from build123d import *

# Parameters (mm, degrees)
SKETCH1_W           = 70
SKETCH1_H           = 70
BOSS_EXTRUDE1_DEPTH = 42
SKETCH2_W           = 70
SKETCH2_H           = 70
BOSS_EXTRUDE2_DEPTH = 6
SKETCH3_R           = 4
CUT_EXTRUDE1_DEPTH  = 74
SKETCH6_W           = 10.07808718
SKETCH6_H           = 10.120371506
SKETCH6_W_2         = 10.137770901
SKETCH6_H_2         = 10.393985643
BOSS_EXTRUDE4_DEPTH = 28
FILLET1_R           = 1
SKETCH4_R           = 4.2
SKETCH4_R_2         = 3
BOSS_EXTRUDE3_DEPTH = 32
CUT_EXTRUDE2_START  = -28
SKETCH8_R           = 3
CUT_EXTRUDE2_DEPTH  = 28
FILLET2_R           = 1


with BuildPart() as part:
    # Sketch1 → Boss-Extrude1 (new body)
    with BuildSketch(Plane(origin=(0, 0, 0), x_dir=(1, 0, 0), z_dir=(0, 1, 0))):
        with Locations((22.315, -31.66)):
            Rectangle(SKETCH1_W, SKETCH1_H)
        with BuildLine():
            Line((1, 0), (43.63, 0))
            ThreePointArc((43.63, 0), (44.337106781, -0.292893219), (44.63, -1))
            Line((44.63, -1), (44.63, -62.32))
            ThreePointArc((44.63, -62.32), (44.337106781, -63.027106781), (43.63, -63.32))
            Line((43.63, -63.32), (1, -63.32))
            ThreePointArc((1, -63.32), (0.292893219, -63.027106781), (0, -62.32))
            Line((0, -62.32), (0, -1))
            ThreePointArc((0, -1), (0.292893219, -0.292893219), (1, 0))
        make_face(mode=Mode.SUBTRACT)
    extrude(amount=BOSS_EXTRUDE1_DEPTH)

    # Sketch2 → Boss-Extrude2 (add)
    with BuildSketch(Plane(origin=(0, 42, 0), x_dir=(1, 0, 0), z_dir=(0, 1, 0))):
        with Locations((22.315, -31.66)):
            Rectangle(SKETCH2_W, SKETCH2_H)
    extrude(amount=BOSS_EXTRUDE2_DEPTH)

    # Sketch3 → Cut-Extrude1 (cut)
    with BuildSketch(Plane.XY.offset(66.66)):
        with Locations((22.315, 33.289388907)):
            Circle(SKETCH3_R)
    extrude(amount=-CUT_EXTRUDE1_DEPTH, mode=Mode.SUBTRACT)

    # Sketch6 → Boss-Extrude4 (add)
    with BuildSketch(Plane(origin=(0, 42, 0), x_dir=(-1, 0, 0), z_dir=(0, -1, 0))):
        with Locations((-5.03904359, -58.259814247)):
            Rectangle(SKETCH6_W, SKETCH6_H)
        with Locations((-39.56111455, -58.259814247)):
            Rectangle(SKETCH6_W_2, SKETCH6_H)
        with Locations((-39.56111455, -5.196992822)):
            Rectangle(SKETCH6_W_2, SKETCH6_H_2)
        with Locations((-5.03904359, -5.196992822)):
            Rectangle(SKETCH6_W, SKETCH6_H_2)
    extrude(amount=BOSS_EXTRUDE4_DEPTH)

    # Fillet1
    fillet1_edges = [part.edges().sort_by_distance(p)[0] for p in [
        (34.492229099, 28, 10.393985643),
        (10.07808718, 28, 10.393985643),
        (10.07808718, 28, 53.199628494),
        (34.492229099, 28, 53.199628494),
    ]]
    fillet(fillet1_edges, radius=FILLET1_R)

    # Sketch4 → Boss-Extrude3 (add)
    # profile 1 of 4: a face of its own
    with BuildSketch(Plane.XZ.offset(-42)):
        with Locations(Location((5.703606864, 5.703606864, 0), (0, 0, 90))):
            Circle(SKETCH4_R)
        with Locations(Location((5.703606864, 5.703606864, 0), (0, 0, 90))):
            Circle(SKETCH4_R_2, mode=Mode.SUBTRACT)
    # profile 2 of 4: a face of its own
    with BuildSketch(Plane.XZ.offset(-42)):
        with Locations(Location((38.926393136, 5.703606864, 0), (0, 0, 270))):
            Circle(SKETCH4_R)
        with Locations(Location((38.926393136, 5.703606864, 0), (0, 0, 270))):
            Circle(SKETCH4_R_2, mode=Mode.SUBTRACT)
    # profile 3 of 4: a face of its own
    with BuildSketch(Plane.XZ.offset(-42)):
        with Locations(Location((38.926393136, 57.616393136, 0), (0, 0, 90))):
            Circle(SKETCH4_R)
        with Locations(Location((38.926393136, 57.616393136, 0), (0, 0, 90))):
            Circle(SKETCH4_R_2, mode=Mode.SUBTRACT)
    # profile 4 of 4: a face of its own
    with BuildSketch(Plane.XZ.offset(-42)):
        with Locations(Location((5.703606864, 57.616393136, 0), (0, 0, 270))):
            Circle(SKETCH4_R)
        with Locations(Location((5.703606864, 57.616393136, 0), (0, 0, 270))):
            Circle(SKETCH4_R_2, mode=Mode.SUBTRACT)
    extrude(amount=BOSS_EXTRUDE3_DEPTH)

    # Sketch8 → Cut-Extrude2 (cut)
    with BuildSketch(Plane(origin=(0, 14, 0), x_dir=(-1, 0, 0), z_dir=(0, -1, 0)).offset(CUT_EXTRUDE2_START)):
        with Locations(Location((-5.703606864, -57.616393136, 0), (0, 0, 90))):
            Circle(SKETCH8_R)
        with Locations(Location((-38.926393136, -57.616393136, 0), (0, 0, 90))):
            Circle(SKETCH8_R)
        with Locations(Location((-38.926393136, -5.703606864, 0), (0, 0, 90))):
            Circle(SKETCH8_R)
        with Locations(Location((-5.703606864, -5.703606864, 0), (0, 0, 90))):
            Circle(SKETCH8_R)
    extrude(amount=CUT_EXTRUDE2_DEPTH, mode=Mode.SUBTRACT)

    # Fillet2
    fillet2_edges = [part.edges().sort_by_distance(p)[0] for p in [
        (18.315, 33.289388907, 0),
        (18.315, 33.289388907, 63.32),
    ]]
    fillet(fillet2_edges, radius=FILLET2_R)


solid = part.part
Build history of the part. All positions in model axes, mm. A direction names the side the tool comes from. Coordinates: 2 decimals unless noted, no trailing zeros. Write each loop counter-clockwise with the first axis right and the second up, starting at its lowest first coordinate (ties: lowest second). Pieces come first, ordered by that corner, then holes. Notation, with made-up numbers: (2.5, 72.25) -> (17.5, 72.25) arc R28 ccw to (17.5, 102.25) -> close; hole circle Ø7 at (-26, 25.25). An arc over 180 degrees is marked (long way). Use CSV: the item, a comma, the result in double quotes. Start each with the question number.
Q1. Cut at A-A, the plane y = 11. State how many separate pieces and enclosed holes the cut face has, then the cut area to 3 significant figures.
Q2. Cut at C-C, the plane x = 12. List the corners of the cut face in (y, z), then the cut area to 3 significant figures.
Q3. Pull direction Y, two halves, no side cores. Call faces 1 (the flat face through (0, 21, 32)), 2 (the flat face through (9, 10, 59)), 3 (the cylindrical face through (19.141, 30.855, -2.154)): released by +Y, released by -Y, zero draft, split by the parting line, or undercut.
Q4. Drill centre lines: probe 1 along Z at (x, y) = (4, 29.5); probe 2 along X at (y, z) = (41, 0.5) (3 decimals); probe 3 along X at (y, z) = (40.5, 18.5) (3 decimals). Where is each one in solid material? Low to high.
Q5. Cut at D-D, the plane y = 22. List the corners of the cut face in (x, z) (3 decimals).
Q6. Cut at B-B, the plane z = 51.5. List the corners of the cut face in (x, y) (3 decimals).
Q7. 3-axis set-ups, long thin cutter, end or side, ignore diameter. For faces 4 (the flat face through (-12.685, 24, 32)), 5 (the flat face through (22, 42, 31)): which of +Z, -Z, +X, -X, +Y, -Y reach the whole face in a straight line?
Q8. Flat gauge pins, fed straight in: pin 1 Ø4 at (x, z) = (6.5, 59) entering from -Y; pin 2 Ø5 at (x, z) = (7, 22) entering from -Y. Where does each tip first touch, or does it go through?
Checked values:
1,separate pieces,"5"
1,enclosed holes,"5"
1,area,"2,180 mm²"
2,outline,"(0, -3.34) -> (48, -3.34) -> (48, 66.66) -> (0, 66.66) -> (0, 63.32) -> (42, 63.32) -> (42, 0) -> (0, 0) -> close"
2,area,"701 mm²"
3,face 1,"zero draft"
3,face 2,"released by -Y"
3,face 3,"undercut"
4,probe 1,"z = -3.34 to 3.23, 8.17 to 10.39, 53.2 to 55.15, 60.09 to 66.66"
4,probe 2,"x = -12.685 to 10.078, 34.492 to 57.315"
4,probe 3,"x = -12.685 to 0, 44.63 to 57.315"
5,outline,"(-12.685, -3.34) -> (57.315, -3.34) -> (57.315, 66.66) -> (-12.685, 66.66) -> close; hole (0, 10.394) -> (9.078, 10.394) arc R1 cw to (10.078, 9.394) -> (10.078, 0) -> (34.492, 0) -> (34.492, 9.394) arc R1 cw to (35.492, 10.394) -> (44.63, 10.394) -> (44.63, 53.2) -> (35.492, 53.2) arc R1 cw to (34.492, 54.2) -> (34.492, 63.32) -> (10.078, 63.32) -> (10.078, 54.2) arc R1 cw to (9.078, 53.2) -> (0, 53.2) -> close; hole circle Ø6 at (5.704, 5.704); hole circle Ø6 at (5.704, 57.616); hole circle Ø6 at (38.926, 5.704); hole circle Ø6 at (38.926, 57.616)"
6,outline,"(-12.685, 0) -> (0, 0) -> (0, 42) -> (44.63, 42) -> (44.63, 0) -> (57.315, 0) -> (57.315, 48) -> (-12.685, 48) -> close"
7,face 4,"+Z, -Z, -X, +Y, -Y"
7,face 5,"-Y"
8,pin 1,"stops at y = 10"
8,pin 2,"stops at y = 42"
